Check sheet for the modelled part. Datum: model origin and axes. Units: mm. Round coordinates to 2 decimals unless told otherwise and drop trailing zeros. Loops run counter-clockwise (first coordinate to the right, second up) from the corner with the lowest first, then second, coordinate; pieces in that order, holes last. Notation, with made-up numbers: (27.25, 30.5) -> (79.25, 30.5) arc R22 cw to (79.25, 40.5) -> close; hole circle Ø11 at (-21, -21). An arc over 180 degrees is marked (long way). Use one line per item in the form item = value. Start each with the question number.
(1) Sectioned sample at B-B (z = 1.2). State how many separate pieces and enclosed holes the cut face has, and give its area (3 significant figures).
(2) Material ranges on probe 1 along Y at (x, z) = (-89, 1.75); probe 2 along Y at (x, z) = (-35, 0.9); probe 3 along X at (y, z) = (35, 0.5), recorded low to high. Write a range as [from, to].
(3) Sectioned sample at A-A (x = -22.5). Record the cut outline in (y, z).
(4) Go/stop test with flat-tipped pins: pin 1 (0.6 mm diameter, centred on x = -70.5, z = 1, fed in from +Y); pin 2 (1 mm diameter, centred on x = 18.5, z = 1.5, fed in from -Y); pin 3 (0.9 mm diameter, centred on x = 14, y = 30, fed in from -Z); pin 4 (1 mm diameter, centred on x = -90.5, z = 0.5, fed in from +Y). Record where each tip stops, or that it passes through.
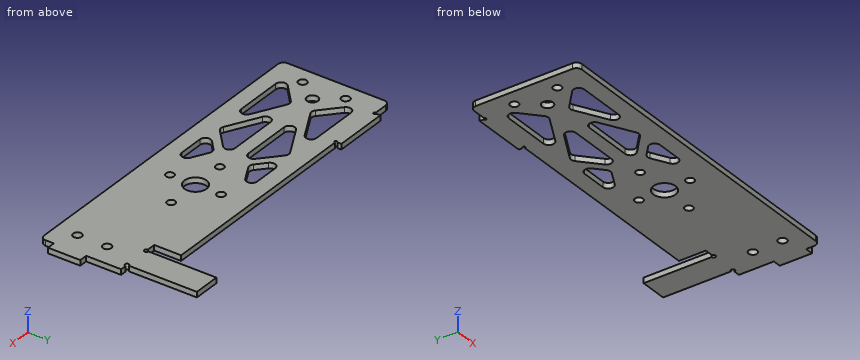
from build123d import *

# Parameters (mm, degrees)
EXTRUDE_1_DEPTH      = 2
SKETCH_2_R           = 1.6
CUT_EXTRUDE_1_DEPTH  = 3
SKETCH_3_W           = 3
SKETCH_3_H           = 24
SKETCH_3_W_2         = 4
CUT_EXTRUDE_2_DEPTH  = 3
SKETCH_4_W           = 3
SKETCH_4_H           = 12
CUT_EXTRUDE_3_DEPTH  = 3
SKETCH_5_W           = 83
SKETCH_5_H           = 30
EXTRUDE_2_DEPTH      = 2
SKETCH_6_R           = 4.1
CUT_EXTRUDE_4_DEPTH  = 3
SKETCH_7_W           = 83
SKETCH_7_H           = 10
EXTRUDE_4_DEPTH      = 2
SKETCH_8_R           = 1.5
CUT_EXTRUDE_5_DEPTH  = 10
SKETCH_13_W          = 2
SKETCH_13_H          = 40
EXTRUDE_6_DEPTH      = 24
SKETCH_16_R          = 0.75
CUT_EXTRUDE_9_DEPTH  = 3
SKETCH_17_W          = 10
SKETCH_17_H          = 2
EXTRUDE_8_DEPTH      = 2
SKETCH_18_W          = 20
SKETCH_18_H          = 2
EXTRUDE_9_DEPTH      = 2
SKETCH_19_R          = 1.55
SKETCH_19_R_2        = 2.05
CUT_EXTRUDE_10_DEPTH = 10
FILLET_1_R           = 2
CUT_EXTRUDE_11_DEPTH = 10
FILLET_2_R           = 2
SKETCH_22_W          = 3
SKETCH_22_H          = 12
EXTRUDE_10_DEPTH     = 2
SKETCH_23_R          = 0.5
CUT_EXTRUDE_12_DEPTH = 10


with BuildPart() as part:
    # 草图1 → 凸台-拉伸1 (new body)
    with BuildSketch(Plane.XY):
        Polygon((0, 0), (17, 0), (17, 5), (20, 5), (20, 17), (17, 17), (17, 54), (0, 54), align=None)
    extrude(amount=EXTRUDE_1_DEPTH)

    # 草图2 → 切除-拉伸1 (cut, through all)
    with BuildSketch(Plane.XY.offset(2)):
        with Locations((9, 8)):
            Circle(SKETCH_2_R)
        with Locations((9, 19)):
            Circle(SKETCH_2_R)
    extrude(amount=-CUT_EXTRUDE_1_DEPTH, mode=Mode.SUBTRACT)

    # 草图3 → 切除-拉伸2 (cut, through all)
    with BuildSketch(Plane.XY.offset(2)):
        with Locations((15.5, 42)):
            Rectangle(SKETCH_3_W, SKETCH_3_H)
        with Locations((2, 42)):
            Rectangle(SKETCH_3_W_2, SKETCH_3_H)
    extrude(amount=-CUT_EXTRUDE_2_DEPTH, mode=Mode.SUBTRACT)

    # 草图4 → 切除-拉伸3 (cut, through all)
    with BuildSketch(Plane.XY.offset(2)):
        with Locations((18.5, 11)):
            Rectangle(SKETCH_4_W, SKETCH_4_H)
    extrude(amount=-CUT_EXTRUDE_3_DEPTH, mode=Mode.SUBTRACT)

    # 草图5 → 凸台-拉伸2 (add, through all)
    with BuildSketch(Plane.XY.offset(2)):
        with Locations((-41.5, 15)):
            Rectangle(SKETCH_5_W, SKETCH_5_H)
    extrude(amount=-EXTRUDE_2_DEPTH)

    # 草图6 → 切除-拉伸4 (cut, through all)
    with BuildSketch(Plane.XY.offset(2)):
        with Locations((-35, 20)):
            Circle(SKETCH_6_R)
    extrude(amount=-CUT_EXTRUDE_4_DEPTH, mode=Mode.SUBTRACT)

    # 草图7 → 凸台-拉伸4 (add, through all)
    with BuildSketch(Plane.XY.offset(2)):
        with Locations((-41.5, 35)):
            Rectangle(SKETCH_7_W, SKETCH_7_H)
    extrude(amount=-EXTRUDE_4_DEPTH)

    # 草图8 → 切除-拉伸5 (cut)
    with BuildSketch(Plane.XY.offset(2)):
        with Locations((-35, 29.5)):
            Circle(SKETCH_8_R)
        with Locations((-35, 10.5)):
            Circle(SKETCH_8_R)
        with Locations((-47.5, 20)):
            Circle(SKETCH_8_R)
        with Locations((-22.5, 20)):
            Circle(SKETCH_8_R)
    extrude(amount=-CUT_EXTRUDE_5_DEPTH, mode=Mode.SUBTRACT)

    # 草图13 → 凸台-拉伸6 (add)
    with BuildSketch(Plane.ZY.offset(83)):
        with Locations((1, 20)):
            Rectangle(SKETCH_13_W, SKETCH_13_H)
    extrude(amount=EXTRUDE_6_DEPTH)

    # 草图16 → 切除-拉伸9 (cut)
    with BuildSketch(Plane(origin=(0, 0, 0), x_dir=(-1, 0, 0), z_dir=(0, 0, -1))):
        with Locations((-4, 30)):
            Circle(SKETCH_16_R)
        with Locations((-14, 30)):
            Circle(SKETCH_16_R)
    extrude(amount=-CUT_EXTRUDE_9_DEPTH, mode=Mode.SUBTRACT)

    # 草图17 → 凸台-拉伸8 (add)
    with BuildSketch(Plane(origin=(0, 54, 0), x_dir=(1, 0, 0), z_dir=(0, 1, 0))):
        with Locations((9, -1)):
            Rectangle(SKETCH_17_W, SKETCH_17_H)
    extrude(amount=EXTRUDE_8_DEPTH)

    # 草图18 → 凸台-拉伸9 (add)
    with BuildSketch(Plane.XY.offset(2)):
        with Locations((-89.439408026, 41)):
            Rectangle(SKETCH_18_W, SKETCH_18_H)
    extrude(amount=-EXTRUDE_9_DEPTH)

    # 草图19 → 切除-拉伸10 (cut)
    with BuildSketch(Plane.XY.offset(2)):
        with Locations((-101.009408026, 12)):
            Circle(SKETCH_19_R)
        with Locations((-101.009408026, 28)):
            Circle(SKETCH_19_R)
        with Locations((-95.009408026, 20)):
            Circle(SKETCH_19_R_2)
    extrude(amount=-CUT_EXTRUDE_10_DEPTH, mode=Mode.SUBTRACT)

    # 圆角1
    fillet_1_edges = [part.edges().sort_by_distance(p)[0] for p in [
        (-107, 0, 1),
        (-107, 40, 1),
        (17, 0, 1),
    ]]
    fillet(fillet_1_edges, radius=FILLET_1_R)

    # 草图21 → 切除-拉伸11 (cut)
    with BuildSketch(Plane(origin=(0, 0, 0), x_dir=(-1, 0, 0), z_dir=(0, 0, -1))):
        Polygon((100.712510242, 6), (89.209450959, 16.338708626), (69.80722773, 6), align=None)
        Polygon((65.227917011, 6.959193961), (85.009408026, 17.5), (53.5, 17.5), align=None)
        Polygon((61.80722773, 6), (53.43509819, 13.524694584), (39.313817735, 6), align=None)
        Polygon((53.43509819, 26.475305416), (39.313817735, 34), (61.80722773, 34), align=None)
        Polygon((85.009408026, 22.5), (53.5, 22.5), (65.227917011, 33.040806039), align=None)
        Polygon((89.209450959, 23.661291374), (69.80722773, 34), (100.712510242, 34), align=None)
    extrude(amount=-CUT_EXTRUDE_11_DEPTH, mode=Mode.SUBTRACT)

    # 圆角2
    fillet_2_edges = [part.edges().sort_by_distance(p)[0] for p in [
        (-61.80722773, 6, 1),
        (-39.313817735, 6, 1),
        (-53.43509819, 13.524694584, 1),
        (-65.227917011, 6.959193961, 1),
        (-53.5, 17.5, 1),
        (-85.009408026, 17.5, 1),
        (-65.227917011, 33.040806039, 1),
        (-85.009408026, 22.5, 1),
        (-53.5, 22.5, 1),
        (-61.80722773, 34, 1),
        (-53.43509819, 26.475305416, 1),
        (-39.313817735, 34, 1),
        (-100.712510242, 34, 1),
        (-89.209450959, 23.661291374, 1),
        (-69.80722773, 34, 1),
        (-100.712510242, 6, 1),
        (-69.80722773, 6, 1),
        (-89.209450959, 16.338708626, 1),
    ]]
    fillet(fillet_2_edges, radius=FILLET_2_R)

    # 草图22 → 凸台-拉伸10 (add)
    with BuildSketch(Plane.XY.offset(2)):
        with Locations((18.5, 11)):
            Rectangle(SKETCH_22_W, SKETCH_22_H)
    extrude(amount=-EXTRUDE_10_DEPTH)

    # 草图23 → 切除-拉伸12 (cut)
    with BuildSketch(Plane.XY.offset(2)):
        with Locations((-79.439408026, 40)):
            Circle(SKETCH_23_R)
        with Locations((-99.439408026, 40)):
            Circle(SKETCH_23_R)
    extrude(amount=-CUT_EXTRUDE_12_DEPTH, mode=Mode.SUBTRACT)


solid = part.part
Checks:
q1.separate_pieces = 1
q1.enclosed_holes = 16
q1.area = 4,270 mm2
q2.probe_1 = [0, 6], [15.91, 24.09], [34, 42]
q2.probe_2 = [0, 9], [12, 15.9], [24.1, 28], [31, 40]
q2.probe_3 = [-107, 0], [4, 14]
q3.outline = (0, 0) -> (18.5, 0) -> (18.5, 2) -> (0, 2) -> close; (21.5, 0) -> (40, 0) -> (40, 2) -> (21.5, 2) -> close
q4.pin_1 = 40
q4.pin_2 = 5
q4.pin_3 = through
q4.pin_4 = 42
